Verification items for the finished model (mm, model axes). Face numbers are marked on the shaded views. A direction names the side the tool comes from. Round coordinates to 2 decimals unless told otherwise and drop trailing zeros. Write each loop counter-clockwise with the first axis right and the second up, starting at its lowest first coordinate (ties: lowest second). Pieces come first, ordered by that corner, then holes.
from build123d import *

# Parameters (mm, degrees)
F0_W     = 35
F0_H     = 15
F1_DEPTH = 4.5
F2_W     = 15
F2_H     = 1.5
F3_DEPTH = 15.001
F4_R     = 3
F5_DEPTH = 3.5
F6_R     = 1.75
F7_DEPTH = 4.501
F8_SIZE  = 2


with BuildPart() as f1:
    # F0 (on Front) → F1 (new body)
    with BuildSketch(Plane.XZ):
        Rectangle(F0_W, F0_H)
    extrude(amount=F1_DEPTH)

    # F2 (on face) → F3 (cut, through all)
    with BuildSketch(Plane.XY.offset(7.5)):
        with Locations((0, -2.25)):
            Rectangle(F2_W, F2_H)
    extrude(amount=-F3_DEPTH, mode=Mode.SUBTRACT)

    # F4 (on face) → F5 (cut)
    with BuildSketch(Plane.XZ.offset(4.5)):
        with Locations((12.5, -2.5)):
            Circle(F4_R)
        with Locations((-12.5, -2.5)):
            Circle(F4_R)
    extrude(amount=-F5_DEPTH, mode=Mode.SUBTRACT)

    # F6 (on face) → F7 (cut, through all)
    with BuildSketch(Plane.XZ.offset(4.5)):
        with Locations((12.5, -2.5)):
            Circle(F6_R)
        with Locations((-12.5, -2.5)):
            Circle(F6_R)
    extrude(amount=-F7_DEPTH, mode=Mode.SUBTRACT)

    # F8
    f8_edges = [f1.edges().sort_by_distance(p)[0] for p in [
        (-17.5, -2.25, 7.5),
        (17.5, -2.25, 7.5),
        (17.5, -2.25, -7.5),
        (-17.5, -2.25, -7.5),
    ]]
    chamfer(f8_edges, length=F8_SIZE)


solid = f1.part
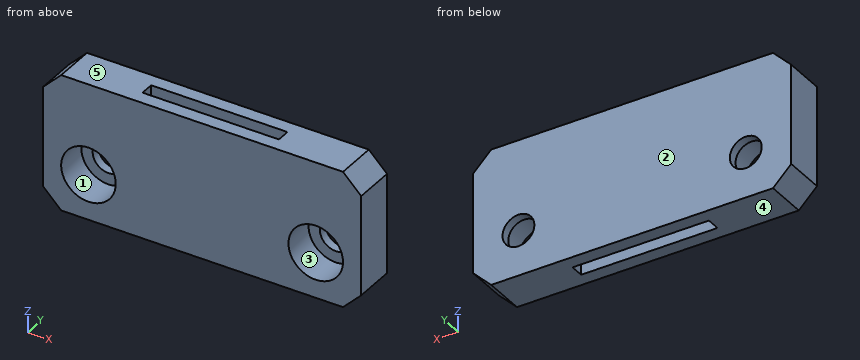
Q1. Sectioned sample at A-A (y = -2.1). Enter the section's corners in (x, z), plus the area to 3 significant figures.
Recorded:
outline: (-17.5, -5.5) - (-15.5, -7.5) - (-7.5, -7.5) - (-7.5, 7.5) - (-15.5, 7.5) - (-17.5, 5.5) - close; (7.5, -7.5) - (15.5, -7.5) - (17.5, -5.5) - (17.5, 5.5) - (15.5, 7.5) - (7.5, 7.5) - close; hole circle Ø6 at (-12.5, -2.5); hole circle Ø6 at (12.5, -2.5)
area: 235 mm2
Q2. Release check for a two-part mould opening along Z. For the marked faces 3, 4 and 5 record: released by +Z, released by -Z, zero draft, split by the parting line, or undercut.
Recorded:
face 3: undercut
face 4: released by -Z
face 5: released by +Z
Q3. Tool access check on the marked faces 1 and 2. Record the directions out of +Z, -Z, +X, -X, +Y, -Y that give a thin tool (end or side, any length) a straight path to the whole face; none if there is none.
Recorded:
face 1: -Y
face 2: +Z, -Z, +X, -X, +Y
Q4. Sectioned sample at C-C (z = 1.5). Enter the section's corners in (x, y), plus the area to 3 significant figures.
Recorded:
outline: (-17.5, -4.5) - (17.5, -4.5) - (17.5, 0) - (-17.5, 0) - close; hole (-7.5, -3) - (7.5, -3) - (7.5, -1.5) - (-7.5, -1.5) - close
area: 135 mm2
Q5. Material ranges on line 1 along Y through (x, z) = (-7, 4.75); line 2 along Z through (x, y) = (-12.5, -2.2); line 3 along Z through (x, y) = (-12.5, -0.5), recorded low to high.
Recorded:
line 1: y = -4.5 to -3, -1.5 to 0
line 2: z = -7.5 to -5.5, 0.5 to 7.5
line 3: z = -7.5 to -4.25, -0.75 to 7.5
Q6. Sectioned sample at B-B (x = 6.5). Enter the section's corners in (y, z).
Recorded:
outline: (-4.5, -7.5) - (-3, -7.5) - (-3, 7.5) - (-4.5, 7.5) - close; (-1.5, -7.5) - (0, -7.5) - (0, 7.5) - (-1.5, 7.5) - close
Q7. Sectioned sample at D-D (y = -3.9). Enter the section's corners in (x, z), plus the area to 3 significant figures.
Recorded:
outline: (-17.5, -5.5) - (-15.5, -7.5) - (15.5, -7.5) - (17.5, -5.5) - (17.5, 5.5) - (15.5, 7.5) - (-15.5, 7.5) - (-17.5, 5.5) - close; hole circle Ø6 at (-12.5, -2.5); hole circle Ø6 at (12.5, -2.5)
area: 460 mm2
